```python
from build123d import *

# Parameters (mm, degrees)
F1_DEPTH = 10
F6_DEPTH = 10


# Not quite as in the source:
# - a feature names something its author has since deleted; it is built from what else it names


with BuildPart() as f1:
    # F0 (on Top) → F1 (new body)
    with BuildSketch(Plane.XY):
        with BuildLine():
            ThreePointArc((-7.0759814838, 3.3989683789), (-6.9640481468, 3.6227797903), (-6.8450379627, 3.8429097425))
            ThreePointArc((-6.8450379627, 3.8429097425), (-7.2244510067, 4.0001671481), (-7.6172716975, 4.1200673333))
            ThreePointArc((-7.6172716975, 4.1200673333), (-7.7361486016, 3.8922728268), (-7.8482152186, 3.6610518743))
            ThreePointArc((-7.8482152186, 3.6610518743), (-7.4549529061, 3.5510643093), (-7.0759814838, 3.3989683789))
        make_face()
        with BuildLine():
            ThreePointArc((-7.6172716975, -4.1200673333), (-7.2244510067, -4.0001671481), (-6.8450379627, -3.8429097425))
            ThreePointArc((-6.8450379627, -3.8429097425), (-6.9640481468, -3.6227797903), (-7.0759814838, -3.3989683789))
            ThreePointArc((-7.0759814838, -3.3989683789), (-7.4549529061, -3.5510643093), (-7.8482152186, -3.6610518743))
            ThreePointArc((-7.8482152186, -3.6610518743), (-7.7361486016, -3.8922728268), (-7.6172716975, -4.1200673333))
        make_face()
        with BuildLine():
            ThreePointArc((-7.8482152186, 3.6610518743), (-7.7361486016, 3.8922728268), (-7.6172716975, 4.1200673333))
            ThreePointArc((-7.6172716975, 4.1200673333), (-12.9101260351, 0), (-7.6172716975, -4.1200673333))
            ThreePointArc((-7.6172716975, -4.1200673333), (-7.7361486016, -3.8922728268), (-7.8482152186, -3.6610518743))
            ThreePointArc((-7.8482152186, -3.6610518743), (-12.4101260351, 0), (-7.8482152186, 3.6610518743))
        make_face()
    extrude(amount=F1_DEPTH)


with BuildPart() as f2_1:
    # F2: copy of F1
    add(f1.part.moved(Location((-14.3, 0, 0))))


with BuildPart() as f3_1:
    # F3: copy of F2_1
    add(f2_1.part.moved(Location((-13, 0, 0))))


with BuildPart() as f1_1:
    add(f1.part)

    # F0 (on Top) → F6 (join)
    with BuildSketch(Plane.XY):
        with BuildLine():
            ThreePointArc((-6.8450379627, 3.8429097425), (0.2165563909, 7.8470123824), (7.0465658628, 3.4595389203))
            Line((7.0465658628, 3.4595389203), (7.0465658628, 5.0342519291))
            ThreePointArc((7.0465658628, 5.0342519291), (-0.5388503097, 8.6433456073), (-7.6172716975, 4.1200673333))
            ThreePointArc((-7.6172716975, 4.1200673333), (-7.2244510067, 4.0001671481), (-6.8450379627, 3.8429097425))
        make_face()
        with BuildLine():
            Line((7.0465658628, -5.0342519291), (7.0465658628, -3.4595389203))
            ThreePointArc((7.0465658628, -3.4595389203), (0.2165563909, -7.8470123824), (-6.8450379627, -3.8429097425))
            ThreePointArc((-6.8450379627, -3.8429097425), (-7.2244510067, -4.0001671481), (-7.6172716975, -4.1200673333))
            ThreePointArc((-7.6172716975, -4.1200673333), (-0.5388503097, -8.6433456073), (7.0465658628, -5.0342519291))
        make_face()
        with BuildLine():
            ThreePointArc((-7.0759814838, 3.3989683789), (-6.9640481468, 3.6227797903), (-6.8450379627, 3.8429097425))
            ThreePointArc((-6.8450379627, 3.8429097425), (-7.2244510067, 4.0001671481), (-7.6172716975, 4.1200673333))
            ThreePointArc((-7.6172716975, 4.1200673333), (-7.7361486016, 3.8922728268), (-7.8482152186, 3.6610518743))
            ThreePointArc((-7.8482152186, 3.6610518743), (-7.4549529061, 3.5510643093), (-7.0759814838, 3.3989683789))
        make_face()
        with BuildLine():
            ThreePointArc((-7.6172716975, -4.1200673333), (-7.2244510067, -4.0001671481), (-6.8450379627, -3.8429097425))
            ThreePointArc((-6.8450379627, -3.8429097425), (-6.9640481468, -3.6227797903), (-7.0759814838, -3.3989683789))
            ThreePointArc((-7.0759814838, -3.3989683789), (-7.4549529061, -3.5510643093), (-7.8482152186, -3.6610518743))
            ThreePointArc((-7.8482152186, -3.6610518743), (-7.7361486016, -3.8922728268), (-7.6172716975, -4.1200673333))
        make_face()
    extrude(amount=F6_DEPTH)


with BuildPart() as f7_1:
    # F7: copy of F1
    add(f1_1.part.moved(Location((-22.5, 0, 0))))


with BuildPart() as f8_1:
    # F8: copy of F1
    add(f1_1.part.moved(Location((0, 18.6, 0))))


with BuildPart() as f9_1:
    # F9: copy of F7_1
    add(f7_1.part.moved(Location((0, 20.1, 0))))


with BuildPart() as f10_1:
    # F10: copy of F7_1
    add(f7_1.part.moved(Location((0, -19.2, 0))))


with BuildPart() as f11_1:
    # F11: copy of F1
    add(f1_1.part.moved(Location((0, -19.5, 0))))


with BuildPart() as f12_1:
    # F12: copy of F1
    add(f1_1.part.moved(Location((25.2, 0, 0))))


solid = f1_1.part
```
Build history of the part. All positions in model axes, mm. Round coordinates to 2 decimals unless told otherwise and drop trailing zeros. Write each loop counter-clockwise with the first axis right and the second up, starting at its lowest first coordinate (ties: lowest second). Pieces come first, ordered by that corner, then holes.
1) Band-saw the part on C-C, the plane z = 3.75. List the corners of the cut face in (x, y).
2) Drill centre lines: probe 1 along Y at (x, z) = (3.75, 7.25); probe 2 along Y at (x, z) = (-7.75, 7); probe 3 along X at (y, z) = (-5.75, 2.75). Where is each one in solid material? Low to high.
3) Band-saw the part on D-D, the plane y = 0. List the corners of the cut face in (x, z), and give its area (3 significant figures).
4) Band-saw the part on A-A, the plane y = 5.5. List the corners of the cut face in (x, z), and give its area (3 significant figures).
5) Band-saw the part on B-B, the plane x = 3.75. List the corners of the cut face in (y, z), and give its area (3 significant figures).
6) Pin check, flat tips, straight feed: pin 1 (5 mm diameter, centred on x = -9.5, z = 8.5, fed in from +Y); pin 2 (1 mm diameter, centred on x = -6.5, z = 5, fed in from -Y); pin 3 (5 mm diameter, centred on y = 3.5, z = 4, fed in from -X); pin 4 (2 mm diameter, centred on x = -7, y = 1.5, fed in from +Z). Stop position of each tip, or through.
Ans:
1. outline: (-7.62, -4.12) arc R8.66 ccw to (7.05, -5.03) - (7.05, -3.46) arc R7.85 cw to (-7.08, -3.4) arc R3.75 cw (long way) to (-7.08, 3.4) arc R7.85 cw to (7.05, 3.46) - (7.05, 5.03) arc R8.66 ccw to (-7.62, 4.12) arc R4.25 ccw (long way) to start
2. probe 1: y = -7.81 to -6.9, 6.9 to 7.81
2. probe 2: y = -4.15 to -3.64, 3.64 to 4.15
2. probe 3: x = -6.48 to -5.34, 5.34 to 6.48
3. outline: (-12.91, 0) - (-12.41, 0) - (-12.41, 10) - (-12.91, 10) - close
3. area: 5.00 mm2
4. outline: (-6.69, 0) - (-5.6, 0) - (-5.6, 10) - (-6.69, 10) - close; (5.6, 0) - (6.69, 0) - (6.69, 10) - (5.6, 10) - close
4. area: 21.8 mm2
5. outline: (-7.81, 0) - (-6.9, 0) - (-6.9, 10) - (-7.81, 10) - close; (6.9, 0) - (7.81, 0) - (7.81, 10) - (6.9, 10) - close
5. area: 18.2 mm2
6. pin 1: stops at y = 5.1
6. pin 2: stops at y = -6.24
6. pin 3: stops at x = -12.79
6. pin 4: passes through
